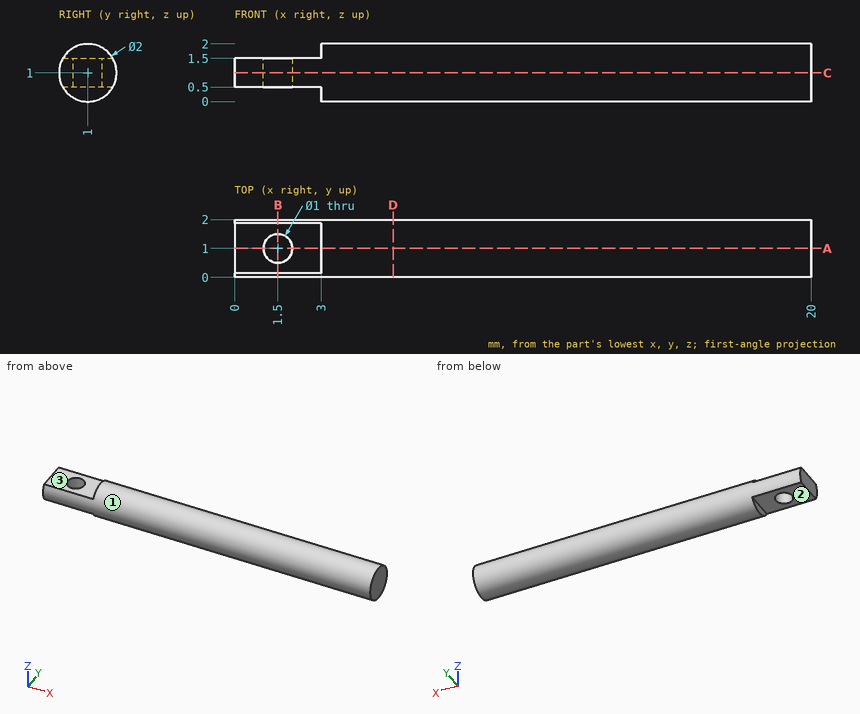
Geometry check sheet. Reference: drawing and pictorial views, mm from the part's lowest x, y, z. A direction names the side the tool comes from. Give positions to 0.01 mm unless a question says otherwise; leave off trailing zeros. Order: outer loops, then holes, each group sorted by start corner. A loop starts at its lowest first (then second) coordinate and runs counter-clockwise, first axis right, second up. Notation, with made-up numbers: M 51.25,41.25 L 76.25,41.25 A28 cw 76.25,69.25 Z; hole C -6,-23.5 d10. An arc over 180 degrees is marked long. Answer in a Markdown table with one row per item. Add a question column.
Q1. Sectioned sample at A-A, the plane y = 1. Record the boundary of the cut face in (x, z).
Q2. Sectioned sample at C-C, the plane z = 1. Record the boundary of the cut face in (x, y).
Q3. Thickness scan on L1, parallel to X at y = 1, z = 1.3; L2, parallel to Z at x = 1, y = 0.65; L3, parallel to Y at x = 1.5, z = 0.95. Record the ranges inside material, lowest first.
Q4. Sectioned sample at D-D, the plane x = 5.5. Record the boundary of the cut face in (y, z), and give its area (3 significant figures).
Q5. Access from +Z, -Z, +X, -X, +Y, -Y to the whole of each face (thin tool, end or side, straight path). Record for the marked faces 1, 2 and 3.
Q6. Sectioned sample at B-B, the plane x = 1.5. Record the boundary of the cut face in (y, z), and give its area (3 significant figures).
Q7. Gauge pin test, flat ends, axial feed: pin 1 Ø0.5 at (x, y) = (2, 1) entering from -Z; pin 2 Ø0.6 at (y, z) = (1, 2) entering from -X. Record the tip position at first contact, or that the pin passes through.
Verdict:
| question | item | result |
|---|---|---|
| 1 | outline | M 0,0.5 L 1,0.5 L 1,1.5 L 0,1.5 Z; M 2,0.5 L 3,0.5 L 3,0 L 20,0 L 20,2 L 3,2 L 3,1.5 L 2,1.5 Z |
| 2 | outline | M 0,0 L 20,0 L 20,2 L 0,2 Z; hole C 1.5,1 d1 |
| 3 | L1 | 0 to 1, 2 to 20 |
| 3 | L2 | 0.5 to 1.5 |
| 3 | L3 | 0 to 0.5, 1.5 to 2 |
| 4 | outline | C 1,1 d2 |
| 4 | area | 3.14 mm² |
| 5 | face 1 | +X, -X |
| 5 | face 2 | -Z, -X, +Y, -Y |
| 5 | face 3 | +Z, -X, +Y, -Y |
| 6 | outline | M 0.13,0.5 L 0.5,0.5 L 0.5,1.5 L 0.13,1.5 A1 ccw Z; M 1.5,0.5 L 1.87,0.5 A1 ccw 1.87,1.5 L 1.5,1.5 Z |
| 6 | area | 0.913 mm² |
| 7 | pin 1 | z = 0.5 |
| 7 | pin 2 | x = 3 |
